For this review, take the finished solid that the model builds, in its own axes (mm). A direction names the side the tool comes from. Coordinates: 2 decimals unless noted, no trailing zeros. Order: outer loops, then holes, each group sorted by start corner. A loop starts at its lowest first (then second) coordinate and runs counter-clockwise, first axis right, second up. Notation, with made-up numbers: (30, -18) - (47, -18) arc R31 cw to (47, 19) - close; hole circle Ø5 at (-12.5, -14.75). An arc over 180 degrees is marked (long way). One line per item, written item: value. Start each with the question number.
(1) For faces 1 (the flat face through (250, 170, 4)), 2 (the flat face through (209, 192, 4)), list the 3-axis set-ups (+Z, -Z, +X, -X, +Y, -Y) from which the entire face can be reached by the end or side of a thin tool; tool diameter is ignored.
(2) Consider section A-A on y = 260. Write out the cut boundary in (x, z), then the cut area to 3 significant figures.
(3) Mouldability with a two-part tool opening along Y and no side actions: class faces 3 (the flat face through (123, 0, 4)), 4 (the flat face through (184, 252, 3.5)), 5 (the flat face through (123, 175, 8)) as released by +Y, released by -Y, zero draft, split by the parting line, or undercut.
(4) To check wall thickness, follow line 1 along Y through (x, z) = (145, 6.8); line 2 along X through (y, z) = (189.5, 2.75); line 3 along X through (y, z) = (278.5, 0.5). State the ranges of each line that lie inside material, in increasing order.
(5) Consider section B-B on z = 5. Write out the cut boundary in (x, y).
Autodesk Inventor part; units mm, degrees
ref_plane "YZ Plane" through (0, 0, 0) normal (1, 0, 0) x (0, 1, 0)
ref_plane "XZ Plane" through (0, 0, 0) normal (0, 1, 0) x (-1, 0, 0)
ref_plane "XY Plane" through (0, 0, 0) normal (0, 0, 1) x (1, 0, 0)
sketch "Sketch1" plane through (0, 0, 0) normal (0, 0, 1) x (1, 0, 0)
  line L0 (0, 0) -> (250, 0)
  line L1 (250, 0) -> (250, 345)
  line L2 (250, 345) -> (0, 345)
  line L3 (0, 345) -> (0, 0)
  dimension "d0" = 250
  dimension "d1" = 345
extrude "Extrusion1" add sketch "Sketch1" along normal blind 8
sketch "Sketch2" plane through (0, 0, 8) normal (0, 0, 1) x (1, 0, 0)
  line L0 (136, 315) -> (230, 315)
  line L1 (230, 315) -> (230, 227)
  line L2 (230, 227) -> (136, 227)
  line L3 (136, 227) -> (136, 315)
  line L4 (250, 0) -> (250, 345)
  line L5 (250, 345) -> (0, 345)
  line L6 (151, 192) -> (162, 192)
  line L7 (162, 192) -> (162, 178)
  line L8 (162, 178) -> (151, 178)
  line L9 (151, 178) -> (151, 192)
  line L10 (204, 192) -> (215, 192)
  line L11 (215, 192) -> (215, 178)
  line L12 (215, 178) -> (204, 178)
  line L13 (204, 178) -> (204, 192)
  circle A0 centre (145, 236) radius 4
  point P0 (0, 0)
  dimension "d4" = 94
  dimension "d5" = 88
  dimension "d6" = 20
  dimension "d7" = 30
  dimension "d8" = 9
  dimension "d9" = 9
  dimension "d10" = 8
  dimension "d11" = 11
  dimension "d12" = 14
  dimension "d13" = 11
  dimension "d14" = 14
  dimension "d15" = 15
  dimension "d16" = 15
  dimension "d17" = 35
extrude "Extrusion2" cut sketch "Sketch2" against normal through all contours L6 L7 L8 L9 | L10 L11 L12 L13 | A0
sketch "Sketch3" plane through (0, 0, 0) normal (0, 0, -1) x (-1, 0, 0)
  line L0 (-230, 315) -> (-136, 315)
  line L1 (-136, 315) -> (-136, 227)
  line L2 (-136, 227) -> (-230, 227)
  line L3 (-230, 227) -> (-230, 315)
  line L4 (-250, 345) -> (0, 345)
  line L5 (-250, 0) -> (-250, 345)
  point P0 (0, 0)
  dimension "d20" = 94
  dimension "d21" = 30
  dimension "d22" = 88
  dimension "d23" = 20
extrude "Extrusion3" cut sketch "Sketch3" against normal blind 3.5
sketch "Sketch4" plane through (0, 0, 3.5) normal (0, 0, -1) x (-1, 0, 0)
  line L0 (-222, 305) -> (-143, 305)
  line L1 (-143, 305) -> (-143, 254)
  line L2 (-143, 254) -> (-222, 254)
  line L3 (-222, 254) -> (-222, 305)
  line L4 (-230, 227) -> (-230, 315)
  line L5 (-136, 315) -> (-136, 227)
  line L6 (-230, 315) -> (-136, 315)
  line L7 (-136, 227) -> (-230, 227)
  point P0 (0, 0)
  dimension "d26" = 8
  dimension "d27" = 7
  dimension "d28" = 10
  dimension "d29" = 27
extrude "Extrusion4" cut sketch "Sketch4" against normal through all contours L0 L1 L2 L3
equation "\"d13\" = d11"
equation "\"d14\" = d12"
properties part number "capac frontal"
Geometry check:
1. face 1: +Z, -Z, +X, +Y, -Y
1. face 2: +Z, -Z
2. outline: (0, 0) - (136, 0) - (136, 3.5) - (143, 3.5) - (143, 8) - (0, 8) - close; (222, 3.5) - (230, 3.5) - (230, 0) - (250, 0) - (250, 8) - (222, 8) - close
2. area: 1,320 mm^2
3. face 3: released by -Y
3. face 4: undercut
3. face 5: zero draft
4. line 1: y = 0 to 232, 240 to 254, 305 to 345
4. line 2: x = 0 to 151, 162 to 204, 215 to 250
4. line 3: x = 0 to 136, 230 to 250
5. outline: (0, 0) - (250, 0) - (250, 345) - (0, 345) - close; hole circle Ø8 at (145, 236); hole (143, 254) - (222, 254) - (222, 305) - (143, 305) - close; hole (151, 178) - (162, 178) - (162, 192) - (151, 192) - close; hole (204, 178) - (215, 178) - (215, 192) - (204, 192) - close
